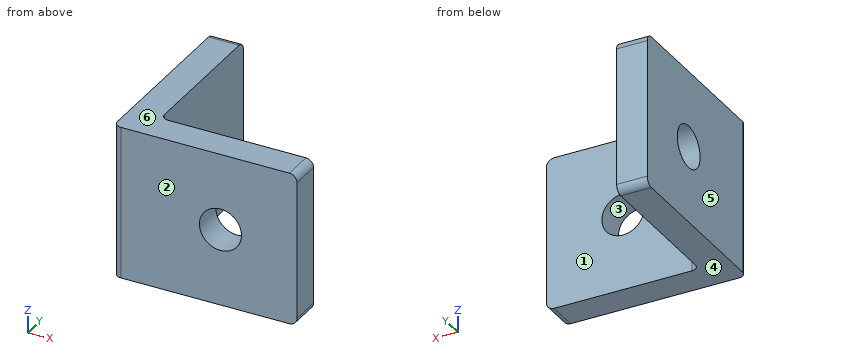
```python
from build123d import *

# Parameters (mm, degrees)
SKETCH_1_W          = 24
SKETCH_1_H          = 4
SKETCH_1_W_2        = 4
SKETCH_1_H_2        = 20
EXTRUDE_1_DEPTH     = 20
SKETCH_2_R          = 2.75
CUT_EXTRUDE_1_DEPTH = 20
SKETCH_3_R          = 2.75
CUT_EXTRUDE_2_DEPTH = 20
FILLET_1_R          = 1


with BuildPart() as part:
    # 스케치1 → 보스-돌출1 (new body)
    with BuildSketch(Plane.XY):
        with Locations((12, -2)):
            Rectangle(SKETCH_1_W, SKETCH_1_H)
        with Locations((2, 10)):
            Rectangle(SKETCH_1_W_2, SKETCH_1_H_2)
    extrude(amount=EXTRUDE_1_DEPTH)

    # 스케치2 → 컷-돌출1 (cut)
    with BuildSketch(Plane(origin=(0, 0, 0), x_dir=(1, 0, 0), z_dir=(0, 1, 0))):
        with Locations(Location((14, -10, 0), (0, 0, 180))):
            Circle(SKETCH_2_R)
    extrude(amount=-CUT_EXTRUDE_1_DEPTH, mode=Mode.SUBTRACT)

    # 스케치3 → 컷-돌출2 (cut)
    with BuildSketch(Plane(origin=(4, 0, 0), x_dir=(0, 0, -1), z_dir=(1, 0, 0))):
        with Locations(Location((-10, 10, 0), (0, 0, 90))):
            Circle(SKETCH_3_R)
    extrude(amount=-CUT_EXTRUDE_2_DEPTH, mode=Mode.SUBTRACT)

    # 필렛1
    fillet_1_edges = [part.edges().sort_by_distance(p)[0] for p in [
        (24, -2, 0),
        (0, -4, 10),
        (4, 0, 10),
        (2, 20, 20),
        (24, -2, 20),
        (2, 20, 0),
    ]]
    fillet(fillet_1_edges, radius=FILLET_1_R)


solid = part.part
```
Check sheet for the modelled part. Datum: model origin and axes. Units: mm. Face numbers are marked on the shaded views. A direction names the side the tool comes from. Coordinates: 2 decimals unless noted, no trailing zeros. Order: outer loops, then holes, each group sorted by start corner. A loop starts at its lowest first (then second) coordinate and runs counter-clockwise, first axis right, second up. Notation, with made-up numbers: (41.5, 25.5) -> (70.5, 25.5) arc R11 ccw to (70.5, 40.5) -> close; hole circle Ø5 at (3, 66.25). An arc over 180 degrees is marked (long way). Write each question's results on one line, items separated by ' | '. Start each with the question number.
1) Draft check along Z on the marked faces 3, 4, 5 and 6. Enter one of: pulls with the +Z half, pulls with the -Z half, needs draft (parallel to the pull), parting line crosses it, or undercut.
2) Depth check by flat-ended pin: pin 1 (1.5 mm diameter, centred on y = 13.5, z = 6.5, fed in from +X); pin 2 (12 mm diameter, centred on y = 1.5, z = 4.5, fed in from +X); pin 3 (8 mm diameter, centred on x = 19, z = 16.5, fed in from +Y). Enter the tip coordinate at first touch or a pass-through.
3) Section check D-D (y = -2.25). Enter the section's corners in (x, z).
4) Material ranges on line 1 along Z through (x, y) = (14, -1.4); line 2 along Y through (x, z) = (5.75, 8.5); line 3 along X through (y, z) = (5.5, 3.5), recorded low to high.
5) Section check B-B (x = 14). Enter the section's corners in (y, z), and give its area (3 significant figures).
6) Section check A-A (z = 10). Enter the section's corners in (x, y), and give its area (3 significant figures).
7) Section check C-C (y = 10). Enter the section's corners in (x, z), and give its area (3 significant figures).
8) Set-up check for the marked faces 1 and 2: record each of +Z, -Z, +X, -X, +Y, -Y from which the full face is reachable in a straight line by a thin tool's end or side.
Checked values:
1) face 3: undercut | face 4: pulls with the -Z half | face 5: needs draft | face 6: pulls with the +Z half
2) pin 1: x = 4 | pin 2: x = 24 | pin 3: y = 0
3) outline: (0, 0) -> (23, 0) arc R1 ccw to (24, 1) -> (24, 19) arc R1 ccw to (23, 20) -> (0, 20) -> close; hole circle Ø5.5 at (14, 10)
4) line 1: 0 to 7.25, 12.75 to 20 | line 2: -4 to 0 | line 3: 0 to 4
5) outline: (-4, 0) -> (0, 0) -> (0, 7.25) -> (-4, 7.25) -> close; (-4, 12.75) -> (0, 12.75) -> (0, 20) -> (-4, 20) -> close | area: 58.0 mm²
6) outline: (0, -3) arc R1 ccw to (1, -4) -> (11.25, -4) -> (11.25, 0) -> (5, 0) arc R1 cw to (4, 1) -> (4, 7.25) -> (0, 7.25) -> close; (0, 12.75) -> (4, 12.75) -> (4, 20) -> (0, 20) -> close; (16.75, -4) -> (24, -4) -> (24, 0) -> (16.75, 0) -> close | area: 132 mm²
7) outline: (0, 0) -> (4, 0) -> (4, 7.25) -> (0, 7.25) -> close; (0, 12.75) -> (4, 12.75) -> (4, 20) -> (0, 20) -> close | area: 58.0 mm²
8) face 1: +Z, -Z, +X, +Y | face 2: +Z, -Z, +X, -X, -Y
